For this review, take the finished solid that the model builds, in its own axes (mm). A direction names the side the tool comes from. Give positions to 0.01 mm unless a question says otherwise; leave off trailing zeros. Write each loop counter-clockwise with the first axis right and the second up, starting at its lowest first coordinate (ties: lowest second). Pieces come first, ordered by that corner, then holes. Notation, with made-up numbers: M 84.25,39 L 109.25,39 A15 ccw 109.25,60 Z; hole C 72.5,55 d5. An arc over 180 degrees is marked long. One line per item, written item: value. Start each with the question number.
Item 1: To check wall thickness, follow probe 1 along Z at (x, y) = (-10.75, 4); probe 2 along X at (y, z) = (4.25, -10.5); probe 3 along Y at (x, z) = (-11.25, -13.5). State the ranges of each line that lie inside material, in increasing order.
Item 2: Consider section B-B, the plane y = 5.5. Write out the cut boundary in (x, z).
Item 3: Consider section D-D, the plane x = 8. Write out the cut boundary in (y, z) (3 decimals).
Item 4: Mouldability with a two-part tool opening along X and no side actions: class faces 1 (the face through (11, 6.35, 12)), 2 (the face through (-9.411, 5, -13)), 3 (the face through (10.586, 1.61, 7.608)) as released by +X, released by -X, zero draft, split by the parting line, or undercut.
Item 5: Clearance check with flat-ended pins moving along their axes: pin 1 Ø1 at (x, y) = (0, 3) entering from -Z; pin 2 Ø7.5 at (x, z) = (-2.5, 4) entering from +Y (3 decimals). State where each tip first meets the part, or that it passes through.
Item 6: Consider section A-A, the plane x = 0. Write out the cut boundary in (y, z) (3 decimals), and give its area (3 significant figures).
Item 7: Tool access review of faces 4 (the face through (10.6, 1.61, -7.63)), 5 (the face through (10.22, 4.78, 8.92)), 6 (the face through (-12, 3, 7.95)): name each direction out of +Z, -Z, +X, -X, +Y, -Y from which nothing blocks a thin tool from reaching the whole face with its end or side.
Item 8: Consider section C-C, the plane z = 1. Write out the cut boundary in (x, y) (3 decimals), and give its area (3 significant figures).
```python
from build123d import *

# Parameters (mm, degrees)
SKETCH1_W                    = 25.4
SKETCH1_H                    = 33.02
BOSS_EXTRUDE1_DEPTH          = 6.35
CUT_EXTRUDE1_REACH           = 37.943
SKETCH2_W                    = 18.8214
SKETCH2_H                    = 3.175
SKETCH3_W                    = 15.9004
SKETCH3_H                    = 3.175
CUT_EXTRUDE2_DEPTH           = 31.952586322
CUT_EXTRUDE3_REACH           = 23.07
SKETCH4_R                    = 6.35
CUT_EXTRUDE4_REACH           = 23.07
CUT_EXTRUDE5_REACH           = 23.07
CUT_EXTRUDE6_DEPTH           = 3.175
F_6_32_TAPPED_HOLE1_D        = 2.7051
F_28_0_1405_DIAMETER_HOLE1_D = 3.5687
F_6_32_TAPPED_HOLE2_REACH    = 32.953
F_6_32_TAPPED_HOLE2_BORE_R   = 1.35255


with BuildPart() as part:
    # Sketch1 → Boss-Extrude1 (new body)
    with BuildSketch(Plane(origin=(0, 0, 0), x_dir=(1, 0, 0), z_dir=(0, 1, 0))):
        Rectangle(SKETCH1_W, SKETCH1_H)
    extrude(amount=BOSS_EXTRUDE1_DEPTH)

    # Sketch2 → Cut-Extrude1 (cut, up to next)
    with BuildSketch(Plane.XY.offset(16.51), mode=Mode.PRIVATE) as cut_extrude1_sk1:
        with Locations((0, 4.7625)):
            Rectangle(SKETCH2_W, SKETCH2_H)
    cut_extrude1_tool1 = extrude(cut_extrude1_sk1.sketch, amount=-CUT_EXTRUDE1_REACH, mode=Mode.PRIVATE) & part.part
    add(cut_extrude1_tool1.solids().sort_by_distance((0, 4.7625, 16.51))[0], mode=Mode.SUBTRACT)

    # Sketch3 → Cut-Extrude2 (cut, through all)
    with BuildSketch(Plane(origin=(12.7, 0, 0), x_dir=(0, 0, -1), z_dir=(1, 0, 0))):
        with Locations((0, 4.7625)):
            Rectangle(SKETCH3_W, SKETCH3_H)
    extrude(amount=-CUT_EXTRUDE2_DEPTH, mode=Mode.SUBTRACT)

    # Sketch4 → Cut-Extrude3 (cut, up to next)
    with BuildSketch(Plane(origin=(0, 3.175, 0), x_dir=(1, 0, 0), z_dir=(0, 1, 0)), mode=Mode.PRIVATE) as cut_extrude3_sk1:
        with Locations(Location((0, 0, 0), (0, 0, 270))):
            Circle(SKETCH4_R)
    cut_extrude3_tool1 = extrude(cut_extrude3_sk1.sketch, amount=-CUT_EXTRUDE3_REACH, mode=Mode.PRIVATE) & part.part
    add(cut_extrude3_tool1.solids().sort_by_distance((0, 3.175, 0))[0], mode=Mode.SUBTRACT)

    # Sketch5 → Cut-Extrude4 (cut, up to next)
    with BuildSketch(Plane(origin=(0, 3.175, 0), x_dir=(-1, 0, 0), z_dir=(0, 1, 0)), mode=Mode.PRIVATE) as cut_extrude4_sk1:
        with BuildLine():
            Line((11.149442765, -7.9502), (12.7, -7.9502))
            Line((12.7, -7.9502), (12.7, 0))
            ThreePointArc((12.7, 0), (12.168507815, -3.635576648), (10.618516919, -6.966857143))
            ThreePointArc((10.618516919, -6.966857143), (10.590684, -7.616884675), (11.149442765, -7.9502))
        make_face()
    cut_extrude4_tool1 = extrude(cut_extrude4_sk1.sketch, amount=-CUT_EXTRUDE4_REACH, mode=Mode.PRIVATE) & part.part
    # Sketch5 → Cut-Extrude4 (cut, up to next)
    with BuildSketch(Plane(origin=(0, 3.175, 0), x_dir=(-1, 0, 0), z_dir=(0, 1, 0)), mode=Mode.PRIVATE) as cut_extrude4_sk2:
        with BuildLine():
            ThreePointArc((10.618516919, 6.966857143), (12.168507815, 3.635576648), (12.7, 0))
            Line((12.7, 0), (12.7, 7.9502))
            Line((12.7, 7.9502), (11.149442765, 7.9502))
            ThreePointArc((11.149442765, 7.9502), (10.590684, 7.616884675), (10.618516919, 6.966857143))
        make_face()
    cut_extrude4_tool2 = extrude(cut_extrude4_sk2.sketch, amount=-CUT_EXTRUDE4_REACH, mode=Mode.PRIVATE) & part.part
    # Sketch5 → Cut-Extrude4 (cut, up to next)
    with BuildSketch(Plane(origin=(0, 3.175, 0), x_dir=(-1, 0, 0), z_dir=(0, 1, 0)), mode=Mode.PRIVATE) as cut_extrude4_sk3:
        with BuildLine():
            ThreePointArc((-10.618516919, -6.966857143), (-12.168507815, -3.635576648), (-12.7, 0))
            Line((-12.7, 0), (-12.7, -7.9502))
            Line((-12.7, -7.9502), (-11.149442765, -7.9502))
            ThreePointArc((-11.149442765, -7.9502), (-10.590684, -7.616884675), (-10.618516919, -6.966857143))
        make_face()
    cut_extrude4_tool3 = extrude(cut_extrude4_sk3.sketch, amount=-CUT_EXTRUDE4_REACH, mode=Mode.PRIVATE) & part.part
    # Sketch5 → Cut-Extrude4 (cut, up to next)
    with BuildSketch(Plane(origin=(0, 3.175, 0), x_dir=(-1, 0, 0), z_dir=(0, 1, 0)), mode=Mode.PRIVATE) as cut_extrude4_sk4:
        with BuildLine():
            Line((-12.7, 7.9502), (-12.7, 0))
            ThreePointArc((-12.7, 0), (-12.168507815, 3.635576648), (-10.618516919, 6.966857143))
            ThreePointArc((-10.618516919, 6.966857143), (-10.590684, 7.616884675), (-11.149442765, 7.9502))
            Line((-11.149442765, 7.9502), (-12.7, 7.9502))
        make_face()
    cut_extrude4_tool4 = extrude(cut_extrude4_sk4.sketch, amount=-CUT_EXTRUDE4_REACH, mode=Mode.PRIVATE) & part.part
    add(cut_extrude4_tool1.solids().sort_by_distance((-11.953453, 3.175, -5.924274))[0], mode=Mode.SUBTRACT)
    add(cut_extrude4_tool2.solids().sort_by_distance((-11.953453, 3.175, 5.924274))[0], mode=Mode.SUBTRACT)
    add(cut_extrude4_tool3.solids().sort_by_distance((11.953453, 3.175, -5.924274))[0], mode=Mode.SUBTRACT)
    add(cut_extrude4_tool4.solids().sort_by_distance((11.953453, 3.175, 5.924274))[0], mode=Mode.SUBTRACT)

    # Sketch6 → Cut-Extrude5 (cut, up to next)
    with BuildSketch(Plane(origin=(0, 3.175, 0), x_dir=(1, 0, 0), z_dir=(0, 1, 0)), mode=Mode.PRIVATE) as cut_extrude5_sk1:
        with BuildLine():
            Line((-9.4107, -10.040384181), (-9.4107, -16.51))
            Line((-9.4107, -16.51), (9.4107, -16.51))
            Line((9.4107, -16.51), (9.4107, -10.040384181))
            ThreePointArc((9.4107, -10.040384181), (9.038249564, -9.462203651), (8.357809524, -9.562270649))
            ThreePointArc((8.357809524, -9.562270649), (0, -12.7), (-8.357809524, -9.562270649))
            ThreePointArc((-8.357809524, -9.562270649), (-9.038249564, -9.462203651), (-9.4107, -10.040384181))
        make_face()
    cut_extrude5_tool1 = extrude(cut_extrude5_sk1.sketch, amount=-CUT_EXTRUDE5_REACH, mode=Mode.PRIVATE) & part.part
    # Sketch6 → Cut-Extrude5 (cut, up to next)
    with BuildSketch(Plane(origin=(0, 3.175, 0), x_dir=(1, 0, 0), z_dir=(0, 1, 0)), mode=Mode.PRIVATE) as cut_extrude5_sk2:
        with BuildLine():
            Line((9.4107, 16.51), (9.4107, 10.040384181))
            ThreePointArc((9.4107, 10.040384181), (9.038249564, 9.462203651), (8.357809524, 9.562270649))
            ThreePointArc((8.357809524, 9.562270649), (0, 12.7), (-8.357809524, 9.562270649))
            ThreePointArc((-8.357809524, 9.562270649), (-9.038249564, 9.462203651), (-9.4107, 10.040384181))
            Line((-9.4107, 10.040384181), (-9.4107, 16.51))
            Line((-9.4107, 16.51), (9.4107, 16.51))
        make_face()
    cut_extrude5_tool2 = extrude(cut_extrude5_sk2.sketch, amount=-CUT_EXTRUDE5_REACH, mode=Mode.PRIVATE) & part.part
    add(cut_extrude5_tool1.solids().sort_by_distance((0, 3.175, 13.865951))[0], mode=Mode.SUBTRACT)
    add(cut_extrude5_tool2.solids().sort_by_distance((0, 3.175, -13.865951))[0], mode=Mode.SUBTRACT)

    # Sketch7 → Cut-Extrude6 (cut)
    with BuildSketch(Plane(origin=(0, 6.35, 0), x_dir=(1, 0, 0), z_dir=(0, 1, 0))):
        Polygon((-11.05535, 7.9502), (-9.4107, 9.8552), (-9.4107, 7.9502), align=None)
        Polygon((-11.05535, -7.9502), (-9.4107, -9.8552), (-9.4107, -7.9502), align=None)
        Polygon((9.4107, -9.8552), (11.05535, -7.9502), (9.4107, -7.9502), align=None)
        Polygon((9.4107, 9.8552), (11.05535, 7.9502), (9.4107, 7.9502), align=None)
    extrude(amount=-CUT_EXTRUDE6_DEPTH, mode=Mode.SUBTRACT)

    # 6-32 Tapped Hole1 (through all)
    with Locations(Plane(origin=(0, 3.175, 0), x_dir=(-1, 0, 0), z_dir=(0, 1, 0))):
        with Locations((0, -9.779), (-9.779, 0), (0, 9.779), (9.779, 0)):
            Hole(F_6_32_TAPPED_HOLE1_D / 2)

    # 28 _0.1405_ Diameter Hole1 (through all)
    with Locations(Plane(origin=(0, 3.175, 0), x_dir=(-1, 0, 0), z_dir=(0, 1, 0))):
        with Locations((6.914797213, -6.914797213), (-6.914797213, -6.914797213), (-6.914797213, 6.914797213), (6.914797213, 6.914797213)):
            Hole(F_28_0_1405_DIAMETER_HOLE1_D / 2)

    # 6-32 Tapped Hole2 bore → 6-32 Tapped Hole2 (cut, up to next)
    with BuildSketch(Plane(origin=(12.7, 0, 0), x_dir=(0, 0, -1), z_dir=(1, 0, 0)), mode=Mode.PRIVATE) as f_6_32_tapped_hole2_sk1:
        with Locations((-13.470384182, 3.175)):
            Circle(F_6_32_TAPPED_HOLE2_BORE_R)
    f_6_32_tapped_hole2_tool1 = extrude(f_6_32_tapped_hole2_sk1.sketch, amount=-F_6_32_TAPPED_HOLE2_REACH, mode=Mode.PRIVATE) & part.part
    # 6-32 Tapped Hole2 bore → 6-32 Tapped Hole2 (cut, up to next)
    with BuildSketch(Plane(origin=(12.7, 0, 0), x_dir=(0, 0, -1), z_dir=(1, 0, 0)), mode=Mode.PRIVATE) as f_6_32_tapped_hole2_sk2:
        with Locations((13.470384182, 3.175)):
            Circle(F_6_32_TAPPED_HOLE2_BORE_R)
    f_6_32_tapped_hole2_tool2 = extrude(f_6_32_tapped_hole2_sk2.sketch, amount=-F_6_32_TAPPED_HOLE2_REACH, mode=Mode.PRIVATE) & part.part
    f_6_32_tapped_hole2_1 = f_6_32_tapped_hole2_tool1.solids().sort_by_distance((12.7, 3.175, 13.470384))[0]
    add(f_6_32_tapped_hole2_1, mode=Mode.SUBTRACT)
    f_6_32_tapped_hole2_2 = f_6_32_tapped_hole2_tool2.solids().sort_by_distance((12.7, 3.175, -13.470384))[0]
    add(f_6_32_tapped_hole2_2, mode=Mode.SUBTRACT)
    f_6_32_tapped_hole2 = f_6_32_tapped_hole2_1 + f_6_32_tapped_hole2_2  # 6-32 Tapped Hole2 as one shape, for the pattern or mirror that repeats it

    # Mirror1: 6-32 Tapped Hole2 across plane
    add(f_6_32_tapped_hole2.mirror(Plane(origin=(0, 0, 0), x_dir=(0, 0, 1), z_dir=(1, 0, 0))), mode=Mode.SUBTRACT)


solid = part.part
```
Model answer:
1. probe 1: z = -16.51 to -14.54, -12.4 to -8.3, 8.3 to 12.4, 14.54 to 16.51
1. probe 2: x = -12.7 to -9.41, 9.41 to 12.7
1. probe 3: y = 0 to 1.82, 4.53 to 6.35
2. outline: M -12.7,-16.51 L -9.41,-16.51 L -9.41,-9.86 L -11.06,-7.95 L -12.7,-7.95 Z; M -12.7,7.95 L -11.06,7.95 L -9.41,9.86 L -9.41,16.51 L -12.7,16.51 Z; M 9.41,-16.51 L 12.7,-16.51 L 12.7,-7.95 L 11.06,-7.95 L 9.41,-9.86 Z; M 9.41,9.86 L 11.06,7.95 L 12.7,7.95 L 12.7,16.51 L 9.41,16.51 Z
3. outline: M 0,-9.864 L 3.175,-9.864 L 3.175,-8.331 L 0,-8.331 Z; M 0,-5.498 L 3.175,-5.498 L 3.175,5.498 L 0,5.498 Z; M 0,8.331 L 3.175,8.331 L 3.175,9.864 L 0,9.864 Z
4. face 1: zero draft
4. face 2: undercut
4. face 3: released by +X
5. pin 1: stops at z = -12.7
5. pin 2: stops at y = 3.175
6. outline: M 0,-12.7 L 3.175,-12.7 L 3.175,-11.132 L 0,-11.132 Z; M 0,-8.426 L 3.175,-8.426 L 3.175,-6.35 L 0,-6.35 Z; M 0,6.35 L 3.175,6.35 L 3.175,8.426 L 0,8.426 Z; M 0,11.132 L 3.175,11.132 L 3.175,12.7 L 0,12.7 Z
6. area: 23.1 mm2
7. face 4: +X, +Y, -Y
7. face 5: +Y
7. face 6: -X, +Y, -Y
8. outline: M -12.661,0 L -10.69,0 L -10.69,3.175 L -12.661,3.175 Z; M -8.868,0 L -6.271,0 L -6.271,3.175 L -8.868,3.175 Z; M 6.271,0 L 8.868,0 L 8.868,3.175 L 6.271,3.175 Z; M 10.69,0 L 12.661,0 L 12.661,3.175 L 10.69,3.175 Z
8. area: 29.0 mm2
